Here's how the part is built. I have some questions about the finished solid (model axes, mm). Face numbers are marked on the shaded views. Coordinates: 2 decimals unless noted, no trailing zeros. Loops run counter-clockwise (first coordinate to the right, second up) from the corner with the lowest first, then second, coordinate; pieces in that order, holes last. Notation, with made-up numbers: (77, 20) - (115, 20) arc R14 cw to (115, 42) - close; hole circle Ø4 at (86.25, -7). An arc over 180 degrees is marked (long way). Use a Markdown table: item, result.
```python
from build123d import *

# Parameters (mm, degrees)
CROQUIS1_R                 = 6
SALIENTE_EXTRUIR1_DEPTH    = 30
CROQUIS2_R                 = 4
CORTAR_EXTRUIR1_DEPTH      = 15
CROQUIS3_W                 = 3.5
CROQUIS3_H                 = 4.242640688
CORTAR_EXTRUIR2_DEPTH      = 7
CORTAR_EXTRUIR3_DEPTH      = 32.176914536
CORTAR_EXTRUIR3_DEPTH_BACK = 32.176914536
CROQUIS4_R                 = 1


with BuildPart() as part:
    # Croquis1 → Saliente-Extruir1 (new body)
    with BuildSketch(Plane.XY):
        Circle(CROQUIS1_R)
    extrude(amount=SALIENTE_EXTRUIR1_DEPTH)

    # Croquis2 → Cortar-Extruir1 (cut)
    with BuildSketch(Plane(origin=(0, 0, 0), x_dir=(-1, 0, 0), z_dir=(0, 0, -1))):
        Circle(CROQUIS2_R)
    extrude(amount=-CORTAR_EXTRUIR1_DEPTH, mode=Mode.SUBTRACT)

    # Croquis3 → Cortar-Extruir2 (cut)
    with BuildSketch(Plane.XY.offset(30)):
        Rectangle(CROQUIS3_W, CROQUIS3_H)
        with BuildLine():
            ThreePointArc((1.75, 2.121320344), (0, 2.75), (-1.75, 2.121320344))
            Line((-1.75, 2.121320344), (1.75, 2.121320344))
        make_face()
        with BuildLine():
            Line((1.75, -2.121320344), (-1.75, -2.121320344))
            ThreePointArc((-1.75, -2.121320344), (0, -2.75), (1.75, -2.121320344))
        make_face()
    extrude(amount=-CORTAR_EXTRUIR2_DEPTH, mode=Mode.SUBTRACT)

    # Croquis4 → Cortar-Extruir3 (cut, two sides: drawn at the far end of the back side and taken through both)
    with BuildSketch(Plane(origin=(0, 0, 0), x_dir=(0, 0, -1), z_dir=(1, 0, 0)).offset(-CORTAR_EXTRUIR3_DEPTH_BACK)):
        with Locations((-8, 0)):
            Circle(CROQUIS4_R)
    extrude(amount=CORTAR_EXTRUIR3_DEPTH + CORTAR_EXTRUIR3_DEPTH_BACK, mode=Mode.SUBTRACT)


solid = part.part
```
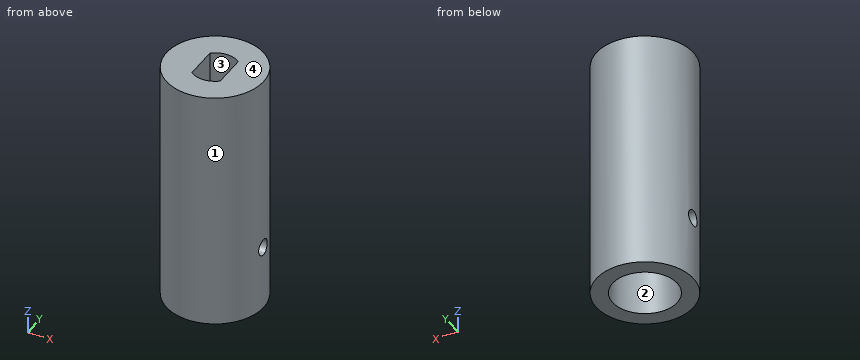
Q1. I want a section at B-B, the plane z = 8. Write out the boundary of the cut face in (x, y), then the cut area to 3 significant figures.
Check values:
| item | result |
|---|---|
| outline | (-5.92, -1) arc R6 ccw to (5.92, -1) - (3.87, -1) arc R4 cw to (-3.87, -1) - close; (-5.92, 1) - (-3.87, 1) arc R4 cw to (3.87, 1) - (5.92, 1) arc R6 ccw to start |
| area | 54.8 mm^2 |
Q2. Please list where these lines run through material, in increasing order: L1, parallel to Z at x = -4.45, y = 0; L2, parallel to Y at x = 0, z = 8.25; L3, parallel to X at y = -0.25, z = 27. Write a range as from..to.
Check values:
| item | result |
|---|---|
| L1 | 0..7, 9..30 |
| L2 | -6..-4, 4..6 |
| L3 | -5.99..-1.75, 1.75..5.99 |
Q3. I want a section at C-C, the plane x = 0. Write out the boundary of the cut face in (y, z).
Check values:
| item | result |
|---|---|
| outline | (-6, 0) - (-4, 0) - (-4, 15) - (4, 15) - (4, 0) - (6, 0) - (6, 30) - (2.75, 30) - (2.75, 23) - (-2.75, 23) - (-2.75, 30) - (-6, 30) - close |
Q4. If we mould it in two halves opening along X, with no side actions, what happens to the marked faces 1, 2, 3 and 4? For each: pulls with the +X half, pulls with the -X half, needs draft (parallel to the pull), parting line crosses it, or undercut.
Check values:
| item | result |
|---|---|
| face 1 | parting line crosses it |
| face 2 | undercut |
| face 3 | undercut |
| face 4 | needs draft |
Q5. I want a section at A-A, the plane y = 0. Write out the boundary of the cut face in (x, z), then the cut area to 4 significant figures.
Check values:
| item | result |
|---|---|
| outline | (-6, 0) - (-4, 0) - (-4, 7) - (-6, 7) - close; (-6, 9) - (-4, 9) - (-4, 15) - (4, 15) - (4, 9) - (6, 9) - (6, 30) - (1.75, 30) - (1.75, 23) - (-1.75, 23) - (-1.75, 30) - (-6, 30) - close; (4, 0) - (6, 0) - (6, 7) - (4, 7) - close |
| area | 207.5 mm^2 |
Q6. I want a section at D-D, the plane y = 1.5. Write out the boundary of the cut face in (x, z), then the cut area to 3 significant figures.
Check values:
| item | result |
|---|---|
| outline | (-5.81, 0) - (-3.71, 0) - (-3.71, 15) - (3.71, 15) - (3.71, 0) - (5.81, 0) - (5.81, 30) - (1.75, 30) - (1.75, 23) - (-1.75, 23) - (-1.75, 30) - (-5.81, 30) - close |
| area | 213 mm^2 |
Q7. Will these pins go through, and if not, where does the flat tip stop? P1, Ø4, axis at x = 2.5, z = 21.5, coming from the +Y side; P2, Ø6.5, axis at x = -0.5, y = 0.5, coming from the -Z side; P3, Ø5, axis at x = 4.5, z = 22.5, coming from the +Y side.
Check values:
| item | result |
|---|---|
| P1 | y = 5.98 |
| P2 | z = 15 |
| P3 | y = 5.66 |
